Could you check a few things on this drawing? It's one solid part, dimensions in mm from its lowest x, y, z. A direction names the side the tool comes from. Give positions to 0.01 mm unless a question says otherwise; leave off trailing zeros. Loops run counter-clockwise (first coordinate to the right, second up) from the corner with the lowest first, then second, coordinate; pieces in that order, holes last.
Q1. Suppose I cut it at D-D (y = 8). List the corners of the cut face in (x, z) for me (1 decimal), and give its area (3 significant figures).
Q2. I'm going to push flat-ended pins straight in: P1, Ø1, axis at y = 6, z = 9, coming from the +X side (1 decimal); P2, Ø1.5, axis at x = 3.5, y = 3.5, coming from the -Z side; P3, Ø5.5, axis at x = 4.25, z = 16, coming from the +Y side; P4, Ø3, axis at x = 16, y = 8, coming from the +Z side. Where does each tip first touch, or does it pass through?
Q3. Suppose I cut it at A-A (x = 16). List the corners of the cut face in (y, z) for me (1 decimal).
Q4. Suppose I cut it at C-C (x = 4.25). List the corners of the cut face in (y, z) for me.
Q5. I need wall thicknesses on probe 1 along X at (y, z) = (1.05, 16); probe 2 along Y at (x, z) = (16, 9.4) (1 decimal); probe 3 along Y at (x, z) = (11, 4). Which ranges of each line are inside material? Lowest first, please.
Q6. For the marked faces 1 and 2, which set-ups out of +Z, -Z, +X, -X, +Y, -Y let a thin tool reach every point of the face, with its end or its side?
Q7. Suppose I cut it at B-B (z = 16). List the corners of the cut face in (x, y) for me, and give its area (3 significant figures).
Q8. Thinking about a two-plate mould opening in Z: for the marked faces 3, 4 and 5, which applies, pulls with the +Z half, pulls with the -Z half, needs draft (parallel to the pull), parting line crosses it, or undercut?
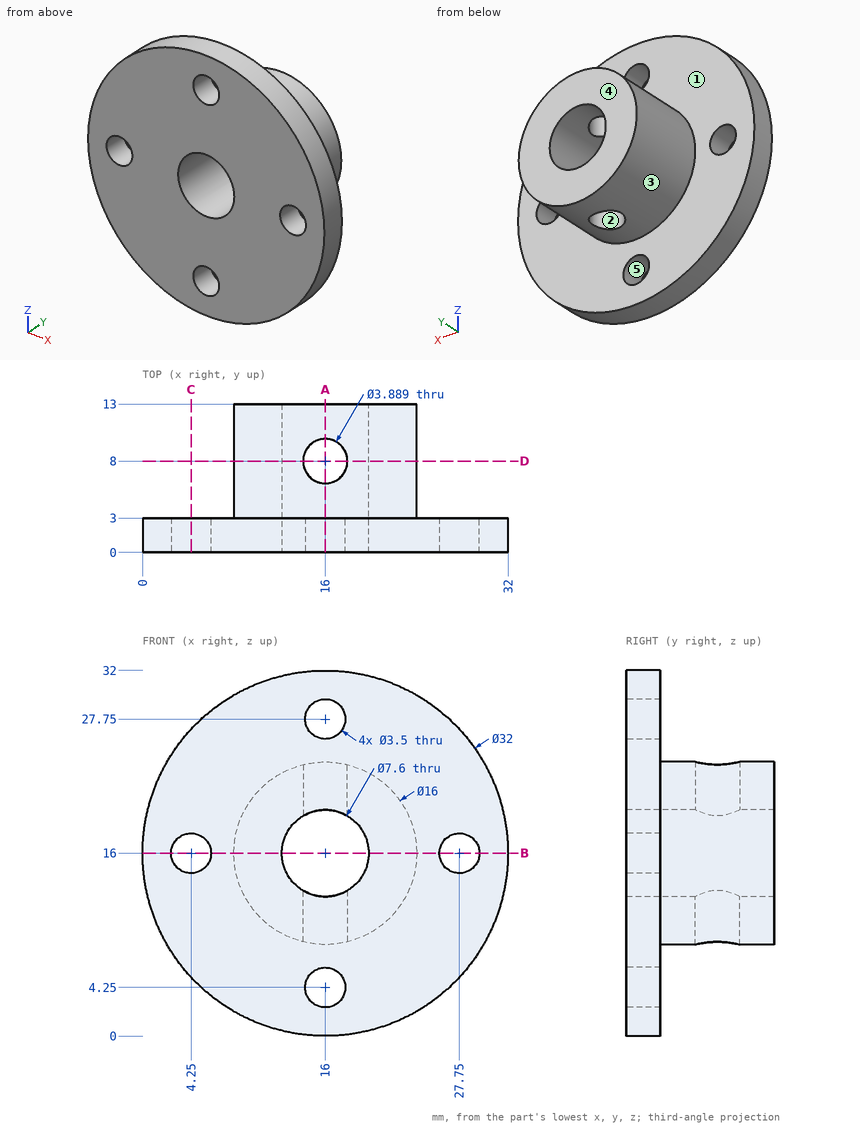
Solutions:
1. outline: (14.1, 8.2) - (14.1, 12.7) arc R3.8 cw to (14.1, 19.3) - (14.1, 23.8) arc R8 ccw to start; (17.9, 8.2) arc R8 ccw to (17.9, 23.8) - (17.9, 19.3) arc R3.8 cw to (17.9, 12.7) - close
1. area: 122 mm2
2. P1: stops at x = 20.7
2. P2: stops at z = 5.35
2. P3: stops at y = 3
2. P4: passes through
3. outline: (0, 0) - (3, 0) - (3, 2.5) - (0, 2.5) - close; (0, 6) - (3, 6) - (3, 8) - (6.1, 8) - (6.1, 12.2) - (0, 12.2) - close; (0, 19.8) - (6.1, 19.8) - (6.1, 24) - (3, 24) - (3, 26) - (0, 26) - close; (0, 29.5) - (3, 29.5) - (3, 32) - (0, 32) - close; (9.9, 8) - (13, 8) - (13, 12.2) - (9.9, 12.2) - close; (9.9, 19.8) - (13, 19.8) - (13, 24) - (9.9, 24) - close
4. outline: (0, 5.14) - (3, 5.14) - (3, 14.25) - (0, 14.25) - close; (0, 17.75) - (3, 17.75) - (3, 26.86) - (0, 26.86) - close
5. probe 1: x = 0 to 2.5, 6 to 12.2, 19.8 to 26, 29.5 to 32
5. probe 2: y = 0 to 6.1, 9.9 to 13
5. probe 3: y = 0 to 3
6. face 1: +Y
6. face 2: +Z, -Z
7. outline: (0, 0) - (2.5, 0) - (2.5, 3) - (0, 3) - close; (6, 0) - (12.2, 0) - (12.2, 13) - (8, 13) - (8, 3) - (6, 3) - close; (19.8, 0) - (26, 0) - (26, 3) - (24, 3) - (24, 13) - (19.8, 13) - close; (29.5, 0) - (32, 0) - (32, 3) - (29.5, 3) - close
7. area: 136 mm2
8. face 3: parting line crosses it
8. face 4: needs draft
8. face 5: undercut
